Verification items for the finished model (mm, model axes). A direction names the side the tool comes from. Give positions to 0.01 mm unless a question says otherwise; leave off trailing zeros. Order: outer loops, then holes, each group sorted by start corner. A loop starts at its lowest first (then second) coordinate and runs counter-clockwise, first axis right, second up.
from build123d import *

# Parameters (mm, degrees)
ESQUISSE1_W             = 300
ESQUISSE1_H             = 30
BOSS_EXTRU_4_DEPTH      = 30
ESQUISSE3_R             = 6
ENL_V_MAT_EXTRU_1_DEPTH = 10


with BuildPart() as part:
    # Esquisse1 → Boss.-Extru.4 (new body)
    with BuildSketch(Plane.XY):
        with Locations((81.373258024, 0.3515625)):
            Rectangle(ESQUISSE1_W, ESQUISSE1_H)
    extrude(amount=BOSS_EXTRU_4_DEPTH)

    # Esquisse3 → Enlèv. mat.-Extru.1 (cut)
    with BuildSketch(Plane.XY):
        with Locations((-53.626741976, 0.3515625)):
            Circle(ESQUISSE3_R)
        with Locations((-23.626741976, 0.3515625)):
            Circle(ESQUISSE3_R)
        with Locations((6.373258024, 0.3515625)):
            Circle(ESQUISSE3_R)
        with Locations((36.373258024, 0.3515625)):
            Circle(ESQUISSE3_R)
        with Locations((66.373258024, 0.3515625)):
            Circle(ESQUISSE3_R)
        with Locations((96.373258024, 0.3515625)):
            Circle(ESQUISSE3_R)
        with Locations((126.373258024, 0.3515625)):
            Circle(ESQUISSE3_R)
        with Locations((156.373258024, 0.3515625)):
            Circle(ESQUISSE3_R)
        with Locations((186.373258024, 0.3515625)):
            Circle(ESQUISSE3_R)
        with Locations((216.373258024, 0.3515625)):
            Circle(ESQUISSE3_R)
    extrude(amount=ENL_V_MAT_EXTRU_1_DEPTH, mode=Mode.SUBTRACT)


solid = part.part
(1) Section check A-A, the plane z = 4.5. Give the number of separate pieces and of enclosed holes in the cut face, then the cut area to 3 significant figures.
Solved:
separate pieces: 1
enclosed holes: 10
area: 7,870 mm2
(2) Scan lines: line 1 (Y direction, x = 37, z = 5.5); line 2 (Z direction, x = 123, y = -3.5); line 3 (Y direction, x = 189, z = 4.5). Record each from-to range of solid material in increasing order.
Solved:
line 1: y = -14.65 to -5.62, 6.32 to 15.35
line 2: z = 10 to 30
line 3: y = -14.65 to -5.04, 5.75 to 15.35
(3) Go/stop test with a flat-tipped pin: pin 1 (3.5 mm diameter, centred on x = 94, y = 3, fed in from -Z). Record where the tip stops, or that it passes through.
Solved:
pin 1: stops at z = 10
(4) Section check B-B, the plane x = 129. Enter the section's corners in (y, z), then the cut area to 3 significant figures.
Solved:
outline: (-14.65, 0) - (-5.04, 0) - (-5.04, 10) - (5.75, 10) - (5.75, 0) - (15.35, 0) - (15.35, 30) - (-14.65, 30) - close
area: 792 mm2
(5) Set-up check for faces 1 (the flat face through (-54, 0, 10)), 2 (the flat face through (231.373, 0, 15)): record each of +Z, -Z, +X, -X, +Y, -Y from which the full face is reachable in a straight line by a thin tool's end or side.
Solved:
face 1: -Z
face 2: +Z, -Z, +X, +Y, -Y
(6) Release check for a two-part mould opening along Y. For faces 3 (the flat face through (79, 1, 0)), 4 (the flat face through (79, -14.648, 15)), 5 (the cylindrical face through (192.096, 2.154, 4.93)), 6 (the flat face through (79, 15.352, 15)) record: pulls with the +Y half, pulls with the -Y half, needs draft (parallel to the pull), parting line crosses it, or undercut.
Solved:
face 3: needs draft
face 4: pulls with the -Y half
face 5: undercut
face 6: pulls with the +Y half
